The listing builds one solid part. Answer for the finished solid, in the listing's coordinates (mm). A direction names the side the tool comes from. Give positions to 0.01 mm unless a question says otherwise; leave off trailing zeros. Order: outer loops, then holes, each group sorted by start corner. A loop starts at its lowest first (then second) coordinate and runs counter-clockwise, first axis right, second up. Notation, with made-up numbers: (18, 50.25) - (76, 50.25) arc R32 cw to (76, 79.25) - close; hole circle Ø2 at (37, -39.5). An arc over 180 degrees is marked (long way). Answer in a Markdown table with one row per item. Add a question column.
```python
from build123d import *

# Parameters (mm, degrees)
BASE_FLANGE1_DEPTH = 8
SKETCH6_R          = 1.5
CUT_EXTRUDE1_DEPTH = 0.7
SKETCH7_R          = 2.15
CUT_EXTRUDE2_DEPTH = 0.7


# Sheet-metal steps are written as plain solids
with BuildPart() as part:
    # Sketch1 → Base-Flange1 (new body)
    with BuildSketch(Plane.XY):
        with BuildLine():
            Line((0, 0), (23.6, 0))
            ThreePointArc((23.6, 0), (24.589949494, 0.410050506), (25, 1.4))
            Line((25, 1.4), (25, 20))
            Line((25, 20), (24.3, 20))
            Line((24.3, 20), (24.3, 1.4))
            ThreePointArc((24.3, 1.4), (24.094974747, 0.905025253), (23.6, 0.7))
            Line((23.6, 0.7), (0, 0.7))
            Line((0, 0.7), (0, 0))
        make_face()
    extrude(amount=BASE_FLANGE1_DEPTH)

    # Sketch6 → Cut-Extrude1 (cut)
    with BuildSketch(Plane(origin=(0, 0.7, 0), x_dir=(1, 0, 0), z_dir=(0, 1, 0))):
        with Locations(Location((7.5, -4, 0), (0, 0, 270))):
            Circle(SKETCH6_R)
        with Locations(Location((17.5, -4, 0), (0, 0, 270))):
            Circle(SKETCH6_R)
    extrude(amount=-CUT_EXTRUDE1_DEPTH, mode=Mode.SUBTRACT)

    # Sketch7 → Cut-Extrude2 (cut)
    with BuildSketch(Plane(origin=(25, 0, 0), x_dir=(0, 0, -1), z_dir=(1, 0, 0))):
        with Locations((-4, 15)):
            Circle(SKETCH7_R)
        with Locations((-4, 5)):
            Circle(SKETCH7_R)
    extrude(amount=-CUT_EXTRUDE2_DEPTH, mode=Mode.SUBTRACT)


solid = part.part
```
(1) Find section C-C, the plane x = 17.5. Write down the section's boundary in (y, z).
(2) Straight lines are drawn through the part: line 1 (Y direction, x = 24.55, z = 4); line 2 (Y direction, x = 11.75, z = 3.5); line 3 (X direction, y = 1.5, z = 7.25). For each, find the intervals that lie inside material, in ascending order.
(3) The mould has two halves that part along X. Classify faces 1 (the face through (18, 0.4, 8)), 2 (the face through (6.17, 0.35, 4.69)), 3 (the face through (25, 11, 4)): +X half, -X half, draft (parallel to the pull), parting line (faces both ways), or undercut.
(4) Find section A-A, the plane y = 15. Write down the section's boundary in (x, z), plus the area to 3 significant figures.
(5) Find section B-B, the plane z = 4. Write down the section's boundary in (x, y).
(6) Find section D-D, the plane y = 11. Write down the section's boundary in (x, z), plus the area to 3 significant figures.
(7) For faces 4 (the face through (18, 0.4, 0)), 5 (the face through (12, 0.7, 4)), determine the directions among +Z, -Z, +X, -X, +Y, -Y from which every point of the face is accessible in a straight line to the end or side of a thin tool.
(8) Each of these flat-tipped pins is pushed along its axis until it touches: P1, Ø2.5, axis at x = 6.5, z = 3, coming from the +Y side; P2, Ø1.8, axis at x = 17.5, z = 4, coming from the +Y side. Where does it stop, or does it pass through?
Answer key:
| question | item | result |
|---|---|---|
| 1 | outline | (0, 0) - (0.7, 0) - (0.7, 2.5) - (0, 2.5) - close; (0, 5.5) - (0.7, 5.5) - (0.7, 8) - (0, 8) - close |
| 2 | line 1 | 0.37 to 2.85, 7.15 to 12.85, 17.15 to 20 |
| 2 | line 2 | 0 to 0.7 |
| 2 | line 3 | 24.3 to 25 |
| 3 | face 1 | draft |
| 3 | face 2 | undercut |
| 3 | face 3 | +X half |
| 4 | outline | (24.3, 0) - (25, 0) - (25, 1.85) - (24.3, 1.85) - close; (24.3, 6.15) - (25, 6.15) - (25, 8) - (24.3, 8) - close |
| 4 | area | 2.59 mm² |
| 5 | outline | (0, 0) - (6, 0) - (6, 0.7) - (0, 0.7) - close; (9, 0) - (16, 0) - (16, 0.7) - (9, 0.7) - close; (19, 0) - (23.6, 0) arc R1.4 ccw to (25, 1.4) - (25, 2.85) - (24.3, 2.85) - (24.3, 1.4) arc R0.7 cw to (23.6, 0.7) - (19, 0.7) - close; (24.3, 7.15) - (25, 7.15) - (25, 12.85) - (24.3, 12.85) - close; (24.3, 17.15) - (25, 17.15) - (25, 20) - (24.3, 20) - close |
| 6 | outline | (24.3, 0) - (25, 0) - (25, 8) - (24.3, 8) - close |
| 6 | area | 5.60 mm² |
| 7 | face 4 | -Z, +X, -X, +Y, -Y |
| 7 | face 5 | +Z, -Z, -X, +Y |
| 8 | P1 | y = 0.7 |
| 8 | P2 | through |
